from build123d import *

# Parameters (mm, degrees)
SKETCH_W      = 300
SKETCH_H      = 300
PAD_DEPTH     = 30
SKETCH001_W   = 300
SKETCH001_H   = 300
SKETCH001_W_2 = 240
SKETCH001_H_2 = 240
PAD001_DEPTH  = 80


with BuildPart() as body:
    # Sketch → Pad (new body)
    with BuildSketch(Plane.XY):
        with Locations((150, 150)):
            Rectangle(SKETCH_W, SKETCH_H)
    extrude(amount=PAD_DEPTH)


with BuildPart() as body001:
    # Sketch001 (on Face6 of Pad) → Pad001 (new body)
    with BuildSketch(Plane.XY.offset(30)):
        with Locations((150, 150)):
            Rectangle(SKETCH001_W, SKETCH001_H)
        with Locations((150, 150)):
            Rectangle(SKETCH001_W_2, SKETCH001_H_2, mode=Mode.SUBTRACT)
    extrude(amount=PAD001_DEPTH)

    # Boolean: union Body
    add(body.part)


solid = body001.part
Geometry: final body of the model. Coordinates: model frame, mm. A direction names the side the tool comes from. Round coordinates to 2 decimals unless told otherwise and drop trailing zeros. Order: outer loops, then holes, each group sorted by start corner. A loop starts at its lowest first (then second) coordinate and runs counter-clockwise, first axis right, second up.
Q1. Material intervals for probe 1 along X at (y, z) = (32, 47); probe 2 along Z at (x, y) = (226, 165), sorted ascending.
Result sheet:
probe 1: x = 0 to 30, 270 to 300
probe 2: z = 0 to 30
Q2. Pin query (flat end, axial travel): pin 1 (1 mm diameter, centred on x = 31.5, y = 47.5, fed in from +Z). Return the tip coordinate at first contact, or that it passes through.
Result sheet:
pin 1: stops at z = 30
Q3. Mould query, pull axis Y, two halves, no side actions, for faces 3 (the face through (0, 148, 54)), 4 (the face through (270, 148, 69)), 5 (the face through (148, 300, 54)). Classes: released by +Y, released by -Y, zero draft, split by the parting line, or undercut.
Result sheet:
face 3: zero draft
face 4: undercut
face 5: released by +Y
Q4. Access query for faces 1 (the face through (148, 152, 30)), 2 (the face through (300, 148, 54)). Directions: +Z, -Z, +X, -X, +Y, -Y. A direction counts if a zero-diameter tool reaches every point of the face in a straight line with its end or side. Return the directions, or none.
Result sheet:
face 1: +Z
face 2: +Z, -Z, +X, +Y, -Y
Q5. Section B-B, the plane x = 156. Output: boundary loops of the cut face in (y, z).
Result sheet:
outline: (0, 0) - (300, 0) - (300, 110) - (270, 110) - (270, 30) - (30, 30) - (30, 110) - (0, 110) - close
Q6. Section A-A, the plane z = 73.5. Output: boundary loops of the cut face in (x, y).
Result sheet:
outline: (0, 0) - (300, 0) - (300, 300) - (0, 300) - close; hole (30, 30) - (270, 30) - (270, 270) - (30, 270) - close
